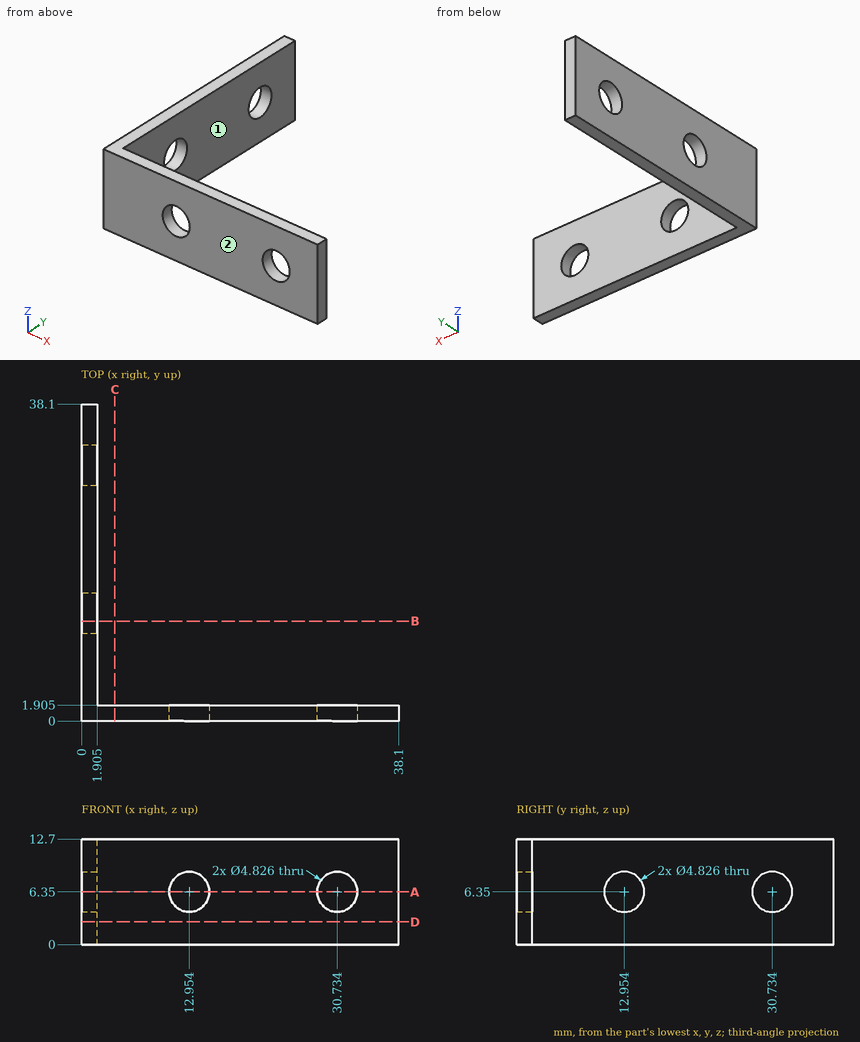
Here's the drawing with two shaded views (mm, measured from the low corner). I have some questions. A direction names the side the tool comes from. Coordinates: 2 decimals unless noted, no trailing zeros. Loops run counter-clockwise (first coordinate to the right, second up) from the corner with the lowest first, then second, coordinate; pieces in that order, holes last. Notation, with made-up numbers: (-14, 80) -> (35, 80) arc R31 ccw to (35, 117) -> close; hole circle Ø1 at (-16.75, 60). An arc over 180 degrees is marked (long way). Answer in a Markdown table with one row per item.
(1) Imagine slicing it at A-A (z = 6.35). List the corners of the cut face in (x, y) for me (3 decimals), plus the area to 3 significant figures.
Results found:
| item | result |
|---|---|
| outline | (0, 0) -> (10.541, 0) -> (10.541, 1.905) -> (1.905, 1.905) -> (1.905, 10.541) -> (0, 10.541) -> close; (0, 15.367) -> (1.905, 15.367) -> (1.905, 28.321) -> (0, 28.321) -> close; (0, 33.147) -> (1.905, 33.147) -> (1.905, 38.1) -> (0, 38.1) -> close; (15.367, 0) -> (28.321, 0) -> (28.321, 1.905) -> (15.367, 1.905) -> close; (33.147, 0) -> (38.1, 0) -> (38.1, 1.905) -> (33.147, 1.905) -> close |
| area | 105 mm^2 |
(2) Will these pins go through, and if not, where does the flat tip stop? pin 1 Ø2 at (x, z) = (30, 9.5) entering from +Y (3 decimals); pin 2 Ø4 at (y, z) = (29, 4.5) entering from +X (3 decimals).
Results found:
| item | result |
|---|---|
| pin 1 | stops at y = 1.905 |
| pin 2 | stops at x = 1.905 |
(3) If I drill on probe 1 along X at (y, z) = (0.7, 6.35); probe 2 along Y at (x, z) = (9.5, 4.75) (3 decimals), over which ranges is the centre line in solid material (lowest first)?
Results found:
| item | result |
|---|---|
| probe 1 | x = 0 to 10.54, 15.37 to 28.32, 33.15 to 38.1 |
| probe 2 | y = 0 to 1.905 |
(4) Imagine slicing it at D-D (z = 2.75). List the corners of the cut face in (x, y) for me (3 decimals), plus the area to 3 significant figures.
Results found:
| item | result |
|---|---|
| outline | (0, 0) -> (38.1, 0) -> (38.1, 1.905) -> (1.905, 1.905) -> (1.905, 38.1) -> (0, 38.1) -> close |
| area | 142 mm^2 |
(5) Imagine slicing it at C-C (x = 4). List the corners of the cut face in (y, z) for me (3 decimals), plus the area to 3 significant figures.
Results found:
| item | result |
|---|---|
| outline | (0, 0) -> (1.905, 0) -> (1.905, 12.7) -> (0, 12.7) -> close |
| area | 24.2 mm^2 |
(6) For the marked faces 1 and 2, which set-ups out of +Z, -Z, +X, -X, +Y, -Y let a thin tool reach every point of the face, with its end or its side?
Results found:
| item | result |
|---|---|
| face 1 | +Z, -Z, +X, +Y |
| face 2 | +Z, -Z, +X, -X, -Y |
(7) Imagine slicing it at B-B (y = 12). List the corners of the cut face in (x, z) for me (3 decimals), plus the area to 3 significant figures.
Results found:
| item | result |
|---|---|
| outline | (0, 0) -> (1.905, 0) -> (1.905, 4.134) -> (0, 4.134) -> close; (0, 8.566) -> (1.905, 8.566) -> (1.905, 12.7) -> (0, 12.7) -> close |
| area | 15.7 mm^2 |
